For this review, take the finished solid that the model builds, in its own axes (mm). Face numbers are marked on the shaded views. A direction names the side the tool comes from. Coordinates: 2 decimals unless noted, no trailing zeros. Loops run counter-clockwise (first coordinate to the right, second up) from the corner with the lowest first, then second, coordinate; pieces in that order, holes last. Notation, with made-up numbers: (1.5, -6) -> (48.5, -6) arc R11 cw to (48.5, 11) -> close; hole circle Ø3 at (-35.75, 75.25). An arc over 180 degrees is marked (long way). One line per item, written item: value.
from build123d import *

# Parameters (mm, degrees)
BOSS_EXTRUDE1_DEPTH = 12.5
SKETCH2_R           = 4.5
SKETCH2_R_2         = 2.5
EXTRUDE_THIN1_DEPTH = 3.5
CUT_EXTRUDE1_REACH  = 30.679
SKETCH3_R           = 2


with BuildPart() as part:
    # Sketch1 → Boss-Extrude1 (new, symmetric)
    with BuildSketch(Plane.XY):
        Polygon((-9, 0), (9, 0), (9, -18.5), (5, -18.5), (5, -4), (-5, -4), (-5, -18.5), (-9, -18.5), align=None)
    extrude(amount=BOSS_EXTRUDE1_DEPTH, both=True)

    # Sketch2 → Extrude-Thin1 (add)
    with BuildSketch(Plane(origin=(0, 0, 0), x_dir=(1, 0, 0), z_dir=(0, 1, 0))):
        Circle(SKETCH2_R)
        Circle(SKETCH2_R_2, mode=Mode.SUBTRACT)
    extrude(amount=EXTRUDE_THIN1_DEPTH)

    # Cut-Extrude1: up to this face of the body (flat: up to its plane)
    cut_extrude1_end = Plane(part.part.faces().sort_by_distance((-9, -9.25, 0))[0])
    # Sketch3 → Cut-Extrude1 (cut, up to the picked face)
    with BuildSketch(Plane(origin=(9, 0, 0), x_dir=(0, 0, -1), z_dir=(1, 0, 0)), mode=Mode.PRIVATE) as cut_extrude1_sk1:
        with Locations((0, -18)):
            Circle(SKETCH3_R)
    cut_extrude1_tool1 = split(extrude(cut_extrude1_sk1.sketch, amount=-CUT_EXTRUDE1_REACH, mode=Mode.PRIVATE), bisect_by=cut_extrude1_end, keep=Keep.BOTH, mode=Mode.PRIVATE)
    add(cut_extrude1_tool1.solids().sort_by(Axis((9, -18, 0), (-1, 0, 0)))[0], mode=Mode.SUBTRACT)


solid = part.part
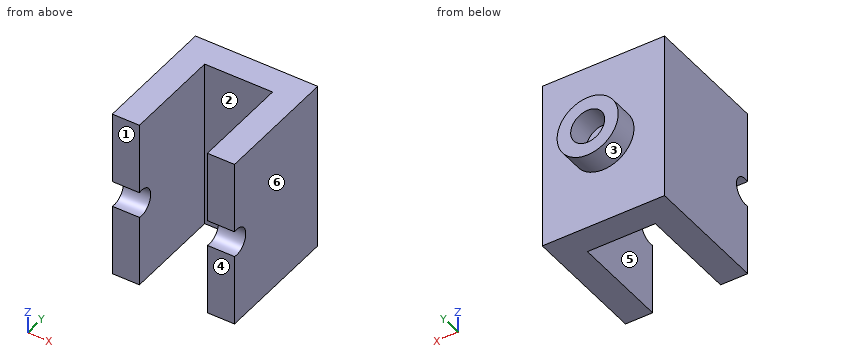
1. Take a section at A-A, the plane y = -8.5. Give the boundary of the cut face in (x, z), and give its area (3 significant figures).
Return value:
outline: (-9, -12.5) -> (-5, -12.5) -> (-5, 12.5) -> (-9, 12.5) -> close; (5, -12.5) -> (9, -12.5) -> (9, 12.5) -> (5, 12.5) -> close
area: 200 mm2
2. To check wall thickness, follow probe 1 along Z at (x, y) = (-6.3, -18); probe 2 along Z at (x, y) = (0, 1.65); probe 3 along X at (y, z) = (-7.5, -9). State the ranges of each line that lie inside material, in increasing order. Write a range as from..to.
Return value:
probe 1: z = -12.5..-2, 2..12.5
probe 2: z = -4.5..-2.5, 2.5..4.5
probe 3: x = -9..-5, 5..9
3. Insertion check: pin 1 Ø3 at (y, z) = (-18, 0) entering from +X; pin 2 Ø1.5 at (x, z) = (2.5, -4) entering from +Y; pin 3 Ø2.5 at (x, z) = (0.5, 1) entering from +Y; pin 4 Ø5 at (x, z) = (1, -0.5) entering from -Y. Each pin has a flat end and moves straight along its axis. Give the tip position at first contact, or say it passes through.
Return value:
pin 1: passes through
pin 2: stops at y = 3.5
pin 3: stops at y = 0
pin 4: stops at y = -4
4. Take a section at D-D, the plane z = 8.25. Give the boundary of the cut face in (x, y), and give its area (3 significant figures).
Return value:
outline: (-9, -18.5) -> (-5, -18.5) -> (-5, -4) -> (5, -4) -> (5, -18.5) -> (9, -18.5) -> (9, 0) -> (-9, 0) -> close
area: 188 mm2
5. The part is to be moulded in two halves that separate along X. For the marked faces 4, 5 and 6, say which applies: pulls with the +X half, pulls with the -X half, needs draft (parallel to the pull), parting line crosses it, or undercut.
Return value:
face 4: needs draft
face 5: undercut
face 6: pulls with the +X half
6. Take a section at B-B, the plane x = 0. Give the boundary of the cut face in (y, z), and give its area (3 significant figures).
Return value:
outline: (-4, -12.5) -> (0, -12.5) -> (0, -4.5) -> (3.5, -4.5) -> (3.5, -2.5) -> (0, -2.5) -> (0, 2.5) -> (3.5, 2.5) -> (3.5, 4.5) -> (0, 4.5) -> (0, 12.5) -> (-4, 12.5) -> close
area: 114 mm2
7. For the marked faces 1, 2 and 3, list the 3-axis set-ups (+Z, -Z, +X, -X, +Y, -Y) from which the entire face can be reached by the end or side of a thin tool; tool diameter is ignored.
Return value:
face 1: +Z, -Z, +X, -X, -Y
face 2: +Z, -Z, -Y
face 3: +Y
8. Take a section at C-C, the plane y = -18. Give the boundary of the cut face in (x, z), and give its area (3 significant figures).
Return value:
outline: (-9, -12.5) -> (-5, -12.5) -> (-5, -2) -> (-9, -2) -> close; (-9, 2) -> (-5, 2) -> (-5, 12.5) -> (-9, 12.5) -> close; (5, -12.5) -> (9, -12.5) -> (9, -2) -> (5, -2) -> close; (5, 2) -> (9, 2) -> (9, 12.5) -> (5, 12.5) -> close
area: 168 mm2
